Verification items for this drawing (mm, ordinates from the low corner). A direction names the side the tool comes from. Coordinates: 2 decimals unless noted, no trailing zeros. Loops run counter-clockwise (first coordinate to the right, second up) from the corner with the lowest first, then second, coordinate; pieces in that order, holes last. Notation, with made-up numbers: M -17.75,-17 L 24.25,-17 A16 cw 24.25,12 Z; hole C -9,87.5 d9. An arc over 180 degrees is marked long. Write each question's results on one line, items separated by ' | '. Start each with the question number.
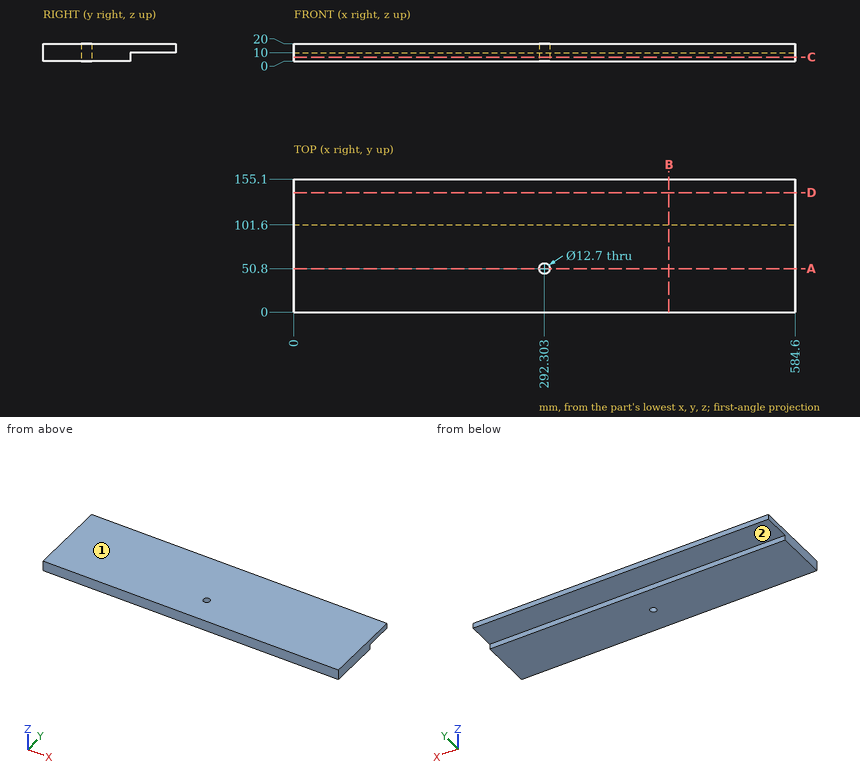
Item 1: Thickness scan on line 1 (X direction, y = 50.8, z = 4); line 2 (Z direction, x = 404, y = 117.5); line 3 (Y direction, x = 330, z = 5). Record the ranges inside material, lowest first.
Item 2: Section check D-D (y = 139.5). Record the cut outline in (x, z), plus the area to 3 significant figures.
Item 3: Section check B-B (x = 437.5). Record the cut outline in (y, z).
Item 4: Section check A-A (y = 50.8). Record the cut outline in (x, z), plus the area to 3 significant figures.
Item 5: Section check C-C (z = 4.75). Record the cut outline in (x, y).
Item 6: Tool access check on the marked faces 1 and 2. Record the directions out of +Z, -Z, +X, -X, +Y, -Y that give a thin tool (end or side, any length) a straight path to the whole face; none if there is none.
Item 7: Depth check by flat-ended pin: P1, Ø16, axis at x = 355, y = 119.5, coming from the -Z side; P2, Ø3, axis at x = 308.5, z = 7, coming from the +Y side. Enter the tip coordinate at first touch or a pass-through.
Computed values:
1) line 1: x = 0 to 285.95, 298.65 to 584.6 | line 2: z = 10 to 20 | line 3: y = 0 to 101.6
2) outline: M 0,10 L 584.6,10 L 584.6,20 L 0,20 Z | area: 5,850 mm²
3) outline: M 0,0 L 101.6,0 L 101.6,10 L 155.1,10 L 155.1,20 L 0,20 Z
4) outline: M 0,0 L 285.95,0 L 285.95,20 L 0,20 Z; M 298.65,0 L 584.6,0 L 584.6,20 L 298.65,20 Z | area: 11,400 mm²
5) outline: M 0,0 L 584.6,0 L 584.6,101.6 L 0,101.6 Z; hole C 292.3,50.8 d12.7
6) face 1: +Z, +X, -X, +Y, -Y | face 2: -Z, +X, -X, +Y
7) P1: stops at z = 10 | P2: stops at y = 101.6
